Input: dimensioned drawing with shaded views. Units: mm. Origin: part minimum x, y, z. A direction names the side the tool comes from. Coordinates: 2 decimals unless noted, no trailing zeros. Order: outer loops, then holes, each group sorted by start corner. A loop starts at its lowest first (then second) coordinate and runs counter-clockwise, first axis right, second up. Notation, with made-up numbers: (88, 10) -> (102, 10) arc R10 cw to (102, 20) -> close; hole circle Ø2 at (25, 29.25). An arc over 180 degrees is marked (long way). Answer as CSV lines item,"result".
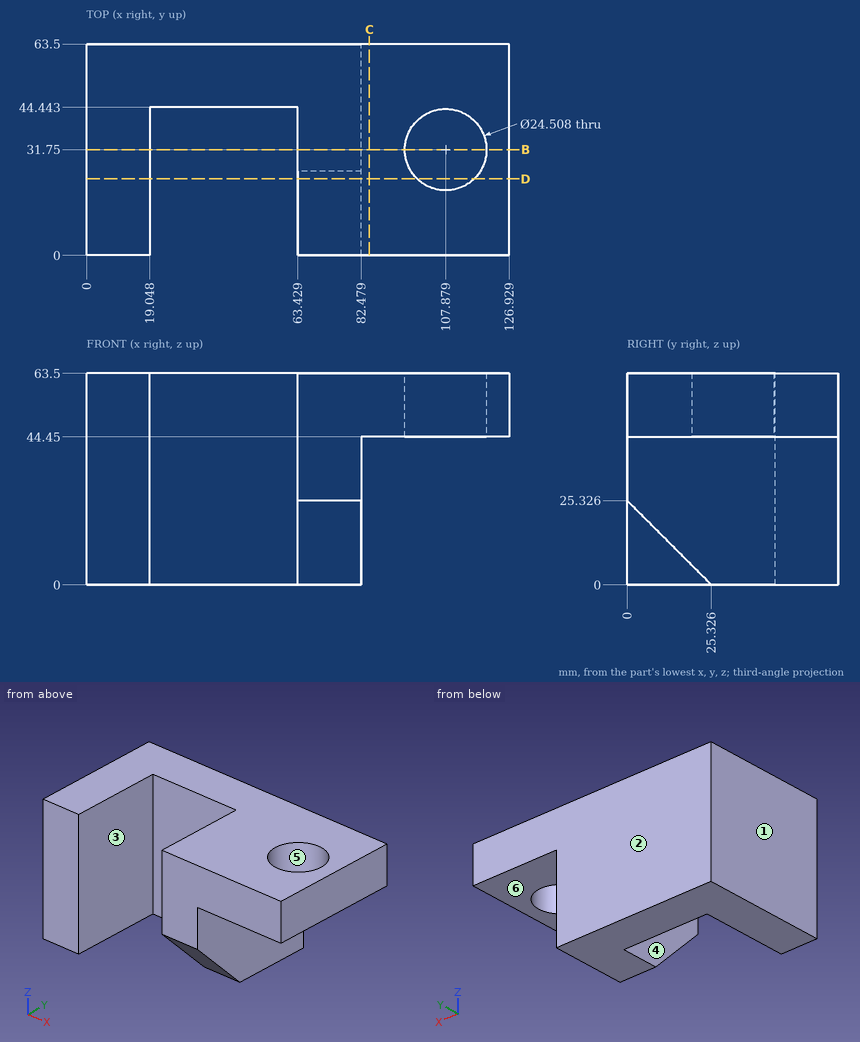
1. Mould query, pull axis X, two halves, no side actions, for the marked faces 1, 2 and 3. Classes: released by +X, released by -X, zero draft, split by the parting line, or undercut.
Findings:
face 1,"released by -X"
face 2,"zero draft"
face 3,"undercut"
2. Cut plane B-B (y = 31.75). State how many separate pieces and enclosed holes the cut face has, plus the area to 3 significant figures.
Findings:
separate pieces,"3"
enclosed holes,"0"
area,"2,800 mm2"
3. Cut plane D-D (y = 23). Return the cut outline in (x, z).
Findings:
outline,"(0, 0) -> (19.05, 0) -> (19.05, 63.5) -> (0, 63.5) -> close; (63.43, 2.33) -> (82.48, 2.33) -> (82.48, 44.45) -> (99.3, 44.45) -> (99.3, 63.5) -> (63.43, 63.5) -> close; (116.46, 44.45) -> (126.93, 44.45) -> (126.93, 63.5) -> (116.46, 63.5) -> close"
4. Ray query, line 1 along X through (y, z) = (17, 18); line 2 along X through (y, z) = (31, 58); line 3 along X through (y, z) = (16, 53). Return the intervals inside material, ascending.
Findings:
line 1,"x = 0 to 19.05, 63.43 to 82.48"
line 2,"x = 0 to 19.05, 63.43 to 95.65, 120.11 to 126.93"
line 3,"x = 0 to 19.05, 63.43 to 126.93"
5. Reachability of the marked faces 4, 5 and 6 from +Z, -Z, +X, -X, +Y, -Y: full face, straight path, thin tool, end or side. Return the list, or none.
Findings:
face 4,"+Z, -Z, -Y"
face 5,"+Z, -Z"
face 6,"-Z, +X, +Y, -Y"
6. Contact query for flat-ended pins moving along their axis: pin 1 (10 mm diameter, centred on x = 50.5, z = 44, fed in from -Y); pin 2 (6 mm diameter, centred on x = 71.5, z = 10, fed in from -Y) (1 decimal); pin 3 (1.5 mm diameter, centred on x = 88, y = 25.5, fed in from -Z). Output: stop coordinate, or through.
Findings:
pin 1,"stops at y = 44.44"
pin 2,"stops at y = 12.3"
pin 3,"stops at z = 44.45"
7. Cut plane C-C (x = 85). Return the cut outline in (y, z).
Findings:
outline,"(0, 44.45) -> (63.5, 44.45) -> (63.5, 63.5) -> (0, 63.5) -> close"
